Geometry check sheet. Reference: the model listing, model coordinates, mm. A direction names the side the tool comes from. Coordinates: 2 decimals unless noted, no trailing zeros. Loops run counter-clockwise (first coordinate to the right, second up) from the corner with the lowest first, then second, coordinate; pieces in that order, holes last.
from build123d import *

# Parameters (mm, degrees)
SKETCH1_W            = 190.5
SKETCH1_H            = 228.6
BOSS_EXTRUDE1_DEPTH  = 6.35
CUT_EXTRUDE1_REACH   = 8.35
SKETCH2_W            = 30.48
SKETCH2_H            = 38.1
BOSS_EXTRUDE2_DEPTH  = 30.48
MIRROR2_COPY_1_DEPTH = 30.48


with BuildPart() as part:
    # Sketch1 → Boss-Extrude1 (new body)
    with BuildSketch(Plane(origin=(0, 0, 0), x_dir=(1, 0, 0), z_dir=(0, 1, 0))):
        Rectangle(SKETCH1_W, SKETCH1_H)
    extrude(amount=BOSS_EXTRUDE1_DEPTH)

    # Sketch2 → Cut-Extrude1 (cut, up to next)
    with BuildSketch(Plane(origin=(0, 6.35, 0), x_dir=(1, 0, 0), z_dir=(0, 1, 0)), mode=Mode.PRIVATE) as cut_extrude1_sk1:
        with Locations((-76.2, 82.55)):
            Rectangle(SKETCH2_W, SKETCH2_H)
    cut_extrude1_tool1 = extrude(cut_extrude1_sk1.sketch, amount=-CUT_EXTRUDE1_REACH, mode=Mode.PRIVATE) & part.part
    add(cut_extrude1_tool1.solids().sort_by_distance((-76.2, 6.35, -82.55))[0], mode=Mode.SUBTRACT)
    # Sketch2 → Cut-Extrude1 (cut, up to next)
    with BuildSketch(Plane(origin=(0, 6.35, 0), x_dir=(1, 0, 0), z_dir=(0, 1, 0)), mode=Mode.PRIVATE) as cut_extrude1_sk2:
        with Locations((-76.2, -82.55)):
            Rectangle(SKETCH2_W, SKETCH2_H)
    cut_extrude1_tool2 = extrude(cut_extrude1_sk2.sketch, amount=-CUT_EXTRUDE1_REACH, mode=Mode.PRIVATE) & part.part
    add(cut_extrude1_tool2.solids().sort_by_distance((-76.2, 6.35, 82.55))[0], mode=Mode.SUBTRACT)
    # Sketch2 → Cut-Extrude1 (cut, up to next)
    with BuildSketch(Plane(origin=(0, 6.35, 0), x_dir=(1, 0, 0), z_dir=(0, 1, 0)), mode=Mode.PRIVATE) as cut_extrude1_sk3:
        with Locations((76.2, -82.55)):
            Rectangle(SKETCH2_W, SKETCH2_H)
    cut_extrude1_tool3 = extrude(cut_extrude1_sk3.sketch, amount=-CUT_EXTRUDE1_REACH, mode=Mode.PRIVATE) & part.part
    add(cut_extrude1_tool3.solids().sort_by_distance((76.2, 6.35, 82.55))[0], mode=Mode.SUBTRACT)
    # Sketch2 → Cut-Extrude1 (cut, up to next)
    with BuildSketch(Plane(origin=(0, 6.35, 0), x_dir=(1, 0, 0), z_dir=(0, 1, 0)), mode=Mode.PRIVATE) as cut_extrude1_sk4:
        with Locations((76.2, 82.55)):
            Rectangle(SKETCH2_W, SKETCH2_H)
    cut_extrude1_tool4 = extrude(cut_extrude1_sk4.sketch, amount=-CUT_EXTRUDE1_REACH, mode=Mode.PRIVATE) & part.part
    add(cut_extrude1_tool4.solids().sort_by_distance((76.2, 6.35, -82.55))[0], mode=Mode.SUBTRACT)

    # Sketch3 → Boss-Extrude2 (add)
    with BuildSketch(Plane.ZY.offset(-91.44)):
        Polygon((-101.6, 6.35), (-101.6, 0), (-99.06, 0), align=None)
    boss_extrude2 = extrude(amount=BOSS_EXTRUDE2_DEPTH)

    # Mirror1: Boss-Extrude2 across plane
    add(boss_extrude2.mirror(Plane.XY))

    # Mirror2: Boss-Extrude2 across plane
    add(boss_extrude2.mirror(Plane(origin=(0, 0, 0), x_dir=(0, 0, 1), z_dir=(1, 0, 0))))

    # Mirror2 copy 1 sketch → Mirror2 copy 1 (add)
    with BuildSketch(Plane(origin=(-91.44, 0, 0), x_dir=(0, 0, -1), z_dir=(1, 0, 0))):
        Polygon((-101.6, 6.35), (-101.6, 0), (-99.06, 0), align=None)
    extrude(amount=MIRROR2_COPY_1_DEPTH)


solid = part.part
(1) Sectioned sample at B-B on y = 4.5. Record the cut outline in (x, z), and give its area (3 significant figures).
Findings:
outline: (-95.25, -114.3) - (95.25, -114.3) - (95.25, 114.3) - (-95.25, 114.3) - close; hole (-91.44, -100.86) - (-60.96, -100.86) - (-60.96, -63.5) - (-91.44, -63.5) - close; hole (-91.44, 63.5) - (-60.96, 63.5) - (-60.96, 100.86) - (-91.44, 100.86) - close; hole (60.96, -100.86) - (91.44, -100.86) - (91.44, -63.5) - (60.96, -63.5) - close; hole (60.96, 63.5) - (91.44, 63.5) - (91.44, 100.86) - (60.96, 100.86) - close
area: 39,000 mm2
(2) Scan lines: L1, parallel to X at y = 5.5, z = -68.5; L2, parallel to Z at x = -71, y = 1.5; L3, parallel to Z at x = -82, y = 0.75. Record each from-to range of solid material in increasing order.
Findings:
L1: x = -95.25 to -91.44, -60.96 to 60.96, 91.44 to 95.25
L2: z = -114.3 to -99.66, -63.5 to 63.5, 99.66 to 114.3
L3: z = -114.3 to -99.36, -63.5 to 63.5, 99.36 to 114.3
(3) Access from +Z, -Z, +X, -X, +Y, -Y to the whole of each face (thin tool, end or side, straight path). Record for faces 1 (the flat face through (-1, 0, 2)), 2 (the flat face through (-76.4, 3.1, -100.3)), 3 (the flat face through (76, 3, -63.5)).
Findings:
face 1: +Z, -Z, +X, -X, -Y
face 2: +Y
face 3: +Y, -Y
(4) Draft check along Z on faces 4 (the flat face through (-91.44, 3, 83)), 5 (the flat face through (-95.25, 3, 2)). Enter one of: +Z half, -Z half, draft (parallel to the pull), parting line (faces both ways), or undercut.
Findings:
face 4: undercut
face 5: draft
(5) Sectioned sample at A-A on z = -69.5. Record the cut outline in (x, y).
Findings:
outline: (-95.25, 0) - (-91.44, 0) - (-91.44, 6.35) - (-95.25, 6.35) - close; (-60.96, 0) - (60.96, 0) - (60.96, 6.35) - (-60.96, 6.35) - close; (91.44, 0) - (95.25, 0) - (95.25, 6.35) - (91.44, 6.35) - close
